Work out the finished part from the listing and answer in its coordinate system (mm). Round coordinates to 2 decimals unless told otherwise and drop trailing zeros. Write each loop counter-clockwise with the first axis right and the second up, starting at its lowest first coordinate (ties: lowest second). Pieces come first, ordered by that corner, then holes. Notation, with made-up numbers: M 11,74 L 59,74 A9 ccw 59,89 Z; hole C 29,10.25 d3. An arc over 180 degrees is marked long. Answer in a Markdown table with one row per item.
Autodesk Inventor part; units mm, degrees
ref_plane "YZ Plane" through (0, 0, 0) normal (1, 0, 0) x (0, 1, 0)
ref_plane "XZ Plane" through (0, 0, 0) normal (0, 1, 0) x (-1, 0, 0)
ref_plane "XY Plane" through (0, 0, 0) normal (0, 0, 1) x (1, 0, 0)
sketch "スケッチ1" plane through (0, 0, 0) normal (1, 0, 0) x (0, 1, 0)
  line L0 (-75, 5) -> (75, 5)
  line L1 (75, 5) -> (75, -5)
  line L2 (75, -5) -> (-75, -5)
  line L3 (-75, -5) -> (-75, 5)
  circle A0 centre (-75, 0) radius 5
  circle A1 centre (75, 0) radius 5
  point P0 (0, 0)
  point P1 (0, 5)
  dimension "d0" = 150
  dimension "d1" = 10
  dimension "d2" = 5
  dimension "d3" = 75
extrude "押し出し1" add sketch "スケッチ1" along normal blind 5 and the other way blind 5 contours A0 L3 | L0 A1 L2 A0 | L1 A1 picked at (-73.4984, 0.7231) picked at (72.0793, -0.9468)
extrude "押し出し2" add sketch "スケッチ1" along normal blind 7.5 and the other way blind 7.5 contours A0 L3 | L3 A0 | A1 L1 | L1 A1
1. The part is cut by section B-B (y = 8.5). Determine the outline of the cut face in (x, z).
Calculated:
| item | result |
|---|---|
| outline | M -5,-5 L 5,-5 L 5,5 L -5,5 Z |
2. Determine the mould class of faces 1 (the cylindrical face through (0.105, 79.619, -1.915)), 2 (the flat face through (7.5, -75, 0)) for opening direction Y: released by +Y, released by -Y, zero draft, split by the parting line, or undercut.
Calculated:
| item | result |
|---|---|
| face 1 | undercut |
| face 2 | zero draft |
3. Given pin 1 (4 mm diameter, centred on x = -1, z = 2.5, fed in from +Y); pin 2 (3 mm diameter, centred on y = -36, z = -2.5, fed in from -X), each flat-ended and moving along its own axis, determine where each tip first touches the part or whether it passes through.
Calculated:
| item | result |
|---|---|
| pin 1 | stops at y = 79.97 |
| pin 2 | stops at x = -5 |
4. The part is cut by section A-A (z = 0). Determine the outline of the cut face in (x, y).
Calculated:
| item | result |
|---|---|
| outline | M -7.5,-80 L 7.5,-80 L 7.5,-70 L 5,-70 L 5,70 L 7.5,70 L 7.5,80 L -7.5,80 L -7.5,70 L -5,70 L -5,-70 L -7.5,-70 Z |
5. Consider line 1 along Y through (x, z) = (6.25, -0.5); line 2 along X through (y, z) = (44.5, -3); line 3 along Y through (x, z) = (3, -0.5). Determine where each line is inside the solid, lowest interval first. Write a range as from..to.
Calculated:
| item | result |
|---|---|
| line 1 | y = -79.97..-70.03, 70.03..79.97 |
| line 2 | x = -5..5 |
| line 3 | y = -79.97..79.97 |
